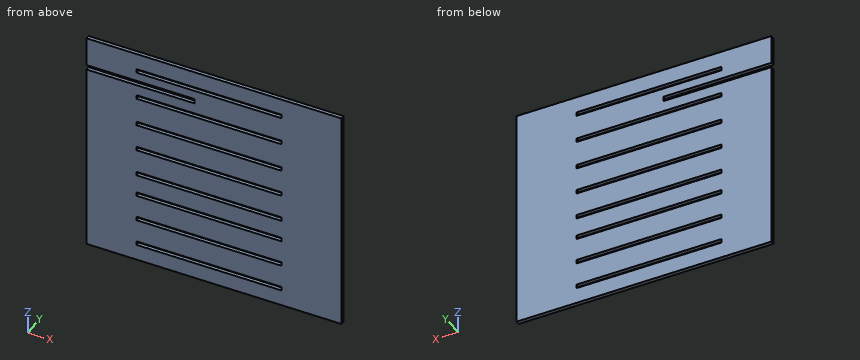
```python
from build123d import *

# Parameters (mm, degrees)
F0_W     = 75
F0_H     = 2
F0_W_2   = 8.9530238211
F0_H_2   = 10.3744039685
F0_H_3   = 13.0056687072
F0_H_4   = 12.9116945341
F1_DEPTH = 1
F2_DEPTH = 2


with BuildPart() as f1:
    # F0 (on Front) → F1 (new body)
    with BuildSketch(Plane.XZ):
        Polygon((-53.6999596655, 0), (-53.6999596655, -10.3744039685), (-6.6999596655, -10.3744039685), (-6.6999596655, -12.8744039685), (-53.6999596655, -12.8744039685), (-62.6529834867, -12.8744039685), (-62.6529834867, -68.3524683118), (69.3470165133, -68.3524683118), (69.3470165133, 48.6475316882), (-62.6529834867, 48.6475316882), (-62.6529834867, 33.4173632413), (-53.6999596655, 33.4173632413), (-6.6999596655, 33.4173632413), (-6.6999596655, 30.9173632413), (-53.6999596655, 30.9173632413), (-53.6999596655, 18.0056687072), (-6.6999596655, 18.0056687072), (-6.6999596655, 15.5056687072), (-53.6999596655, 15.5056687072), (-53.6999596655, 2.5), (-6.6999596655, 2.5), (-6.6999596655, 0), align=None)
        with Locations((0.7488928735, -58.9818040133)):
            Rectangle(F0_W, F0_H, mode=Mode.SUBTRACT)
        with Locations((0.7488928735, -44.9531620145)):
            Rectangle(F0_W, F0_H, mode=Mode.SUBTRACT)
        with Locations((0.7488928735, -31.0450477302)):
            Rectangle(F0_W, F0_H, mode=Mode.SUBTRACT)
        with Locations((0.7488928735, -19.3923042864)):
            Rectangle(F0_W, F0_H, mode=Mode.SUBTRACT)
        with Locations((0.7488928735, -5.1082937755)):
            Rectangle(F0_W, F0_H, mode=Mode.SUBTRACT)
        with Locations((0.7488928735, 9.1280854344)):
            Rectangle(F0_W, F0_H, mode=Mode.SUBTRACT)
        with Locations((0.7488928735, 24.2115164399)):
            Rectangle(F0_W, F0_H, mode=Mode.SUBTRACT)
        with Locations((0.7488928735, 39.0593687296)):
            Rectangle(F0_W, F0_H, mode=Mode.SUBTRACT)
        with Locations((-58.1764715761, -5.1872019842)):
            Rectangle(F0_W_2, F0_H_2)
        Polygon((-6.6999596655, -10.3744039685), (-53.6999596655, -10.3744039685), (-62.6529834867, -10.3744039685), (-62.6529834867, -12.8744039685), (-53.6999596655, -12.8744039685), (-6.6999596655, -12.8744039685), align=None)
        Polygon((-62.6529834867, 0), (-53.6999596655, 0), (-6.6999596655, 0), (-6.6999596655, 2.5), (-53.6999596655, 2.5), (-62.6529834867, 2.5), align=None)
        with Locations((-58.1764715761, 9.0028343536)):
            Rectangle(F0_W_2, F0_H_3)
        Polygon((-62.6529834867, 18.0056687072), (-62.6529834867, 15.5056687072), (-53.6999596655, 15.5056687072), (-6.6999596655, 15.5056687072), (-6.6999596655, 18.0056687072), (-53.6999596655, 18.0056687072), align=None)
        with Locations((-58.1764715761, 24.4615159743)):
            Rectangle(F0_W_2, F0_H_4)
    extrude(amount=F1_DEPTH)

    # F0 (on Front) → F2 (join)
    with BuildSketch(Plane.XZ):
        Polygon((-53.6999596655, 0), (-53.6999596655, -10.3744039685), (-6.6999596655, -10.3744039685), (-6.6999596655, -12.8744039685), (-53.6999596655, -12.8744039685), (-62.6529834867, -12.8744039685), (-62.6529834867, -68.3524683118), (69.3470165133, -68.3524683118), (69.3470165133, 48.6475316882), (-62.6529834867, 48.6475316882), (-62.6529834867, 33.4173632413), (-53.6999596655, 33.4173632413), (-6.6999596655, 33.4173632413), (-6.6999596655, 30.9173632413), (-53.6999596655, 30.9173632413), (-53.6999596655, 18.0056687072), (-6.6999596655, 18.0056687072), (-6.6999596655, 15.5056687072), (-53.6999596655, 15.5056687072), (-53.6999596655, 2.5), (-6.6999596655, 2.5), (-6.6999596655, 0), align=None)
        with Locations((0.7488928735, -58.9818040133)):
            Rectangle(F0_W, F0_H, mode=Mode.SUBTRACT)
        with Locations((0.7488928735, -44.9531620145)):
            Rectangle(F0_W, F0_H, mode=Mode.SUBTRACT)
        with Locations((0.7488928735, -31.0450477302)):
            Rectangle(F0_W, F0_H, mode=Mode.SUBTRACT)
        with Locations((0.7488928735, -19.3923042864)):
            Rectangle(F0_W, F0_H, mode=Mode.SUBTRACT)
        with Locations((0.7488928735, -5.1082937755)):
            Rectangle(F0_W, F0_H, mode=Mode.SUBTRACT)
        with Locations((0.7488928735, 9.1280854344)):
            Rectangle(F0_W, F0_H, mode=Mode.SUBTRACT)
        with Locations((0.7488928735, 24.2115164399)):
            Rectangle(F0_W, F0_H, mode=Mode.SUBTRACT)
        with Locations((0.7488928735, 39.0593687296)):
            Rectangle(F0_W, F0_H, mode=Mode.SUBTRACT)
        with Locations((-58.1764715761, -5.1872019842)):
            Rectangle(F0_W_2, F0_H_2)
        Polygon((-6.6999596655, -10.3744039685), (-53.6999596655, -10.3744039685), (-62.6529834867, -10.3744039685), (-62.6529834867, -12.8744039685), (-53.6999596655, -12.8744039685), (-6.6999596655, -12.8744039685), align=None)
        Polygon((-62.6529834867, 0), (-53.6999596655, 0), (-6.6999596655, 0), (-6.6999596655, 2.5), (-53.6999596655, 2.5), (-62.6529834867, 2.5), align=None)
        with Locations((-58.1764715761, 9.0028343536)):
            Rectangle(F0_W_2, F0_H_3)
        Polygon((-62.6529834867, 18.0056687072), (-62.6529834867, 15.5056687072), (-53.6999596655, 15.5056687072), (-6.6999596655, 15.5056687072), (-6.6999596655, 18.0056687072), (-53.6999596655, 18.0056687072), align=None)
        with Locations((-58.1764715761, 24.4615159743)):
            Rectangle(F0_W_2, F0_H_4)
    extrude(amount=F2_DEPTH)


solid = f1.part
```
The model under review builds one solid part; all positions refer to its coordinate system, in mm. Give positions to 0.01 mm unless a question says otherwise; leave off trailing zeros. Write each loop counter-clockwise with the first axis right and the second up, starting at its lowest first coordinate (ties: lowest second). Pieces come first, ordered by that corner, then holes. Notation, with made-up numbers: (16.25, -11.5) -> (42.25, -11.5) arc R13 cw to (42.25, 3.5) -> close; hole circle Ø2 at (51.5, 43.25). An arc over 180 degrees is marked (long way). Answer in a Markdown table with one row per item.
1) For L1, parallel to X at y = -1.85, z = -6; L2, parallel to Z at x = -52.5, y = -0.75, list the stretches that pass through material, from the lowest coordinate up. Write a range as [from, to].
Worked answers:
| item | result |
|---|---|
| L1 | [-62.65, -36.75], [38.25, 69.35] |
| L2 | [-68.35, 30.92], [33.42, 48.65] |
2) Add section B-B on x = 15. Count the separate pieces of the cut face and the enclosed holes in it, plus the area to 3 significant figures.
Worked answers:
| item | result |
|---|---|
| separate pieces | 9 |
| enclosed holes | 0 |
| area | 202 mm² |
3) Add section A-A on x = -38.5. State the section outline as (y, z) points, plus the area to 3 significant figures.
Worked answers:
| item | result |
|---|---|
| outline | (-2, -68.35) -> (0, -68.35) -> (0, 30.92) -> (-2, 30.92) -> close; (-2, 33.42) -> (0, 33.42) -> (0, 48.65) -> (-2, 48.65) -> close |
| area | 229 mm² |
